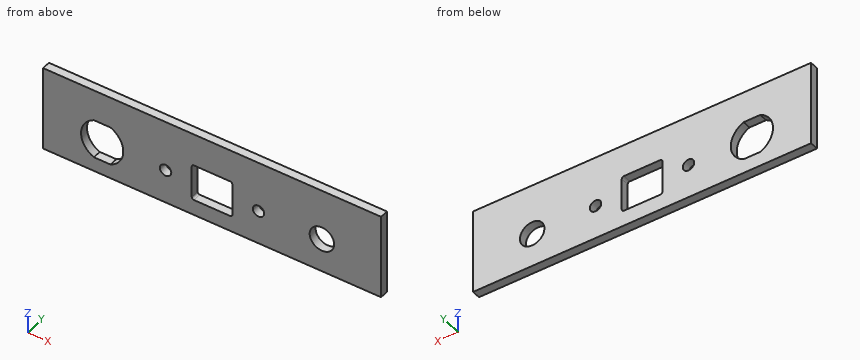
```python
from build123d import *

# Parameters (mm, degrees)
F0_W     = 101.6
F0_H     = 25.4
F1_DEPTH = 2.54
F2_R     = 1.7145
F2_R_2   = 3.683
F3_DEPTH = 2.541


with BuildPart() as f1:
    # F0 (on Front) → F1 (new body)
    with BuildSketch(Plane.XZ):
        with Locations((0, 2.54)):
            Rectangle(F0_W, F0_H)
    extrude(amount=-F1_DEPTH)

    # F2 (on face) → F3 (cut, through all)
    with BuildSketch(Plane.XZ):
        with BuildLine():
            Line((-30.531318, 5.842), (-35.508682, 5.842))
            ThreePointArc((-35.508682, 5.842), (-39.37, 0), (-35.508682, -5.842))
            Line((-35.508682, -5.842), (-30.531318, -5.842))
            ThreePointArc((-30.531318, -5.842), (-26.67, 0), (-30.531318, 5.842))
        make_face()
        with Locations((-13.97, 0)):
            Circle(F2_R)
        with Locations((13.97, 0)):
            Circle(F2_R)
        with Locations((33.02, 0)):
            Circle(F2_R_2)
        with BuildLine():
            ThreePointArc((6.096, 4.826), (5.910013, 5.275013), (5.461, 5.461))
            Line((5.461, 5.461), (-5.461, 5.461))
            ThreePointArc((-5.461, 5.461), (-5.910013, 5.275013), (-6.096, 4.826))
            Line((-6.096, 4.826), (-6.096, -4.826))
            ThreePointArc((-6.096, -4.826), (-5.910013, -5.275013), (-5.461, -5.461))
            Line((-5.461, -5.461), (5.461, -5.461))
            ThreePointArc((5.461, -5.461), (5.910013, -5.275013), (6.096, -4.826))
            Line((6.096, -4.826), (6.096, 4.826))
        make_face()
    extrude(amount=-F3_DEPTH, mode=Mode.SUBTRACT)


solid = f1.part
```
Source: CAD feature listing. Evaluate the final solid. Frame: model axes, mm. Give positions to 0.01 mm unless a question says otherwise; leave off trailing zeros. Loops run counter-clockwise (first coordinate to the right, second up) from the corner with the lowest first, then second, coordinate; pieces in that order, holes last. Notation, with made-up numbers: (-14, -30) -> (23, -30) arc R25 cw to (23, 6) -> close; hole circle Ø4 at (-9.75, 0.25). An arc over 180 degrees is marked (long way). Use a Markdown table: item, result. Add a question column.
(1) Section query C-C (y = 0.45). Count the separate pieces of the cut face and the enclosed holes in it, then the cut area to 3 significant figures.
(2) Ray query, line 1 (X direction, y = 1.95, z = -0.25); line 2 (Z direction, x = -33, y = 2.4); line 3 (Z direction, x = 13.97, y = 2.05). Return the intervals inside material, ascending.
(3) Section query A-A (x = 13.97). Output: boundary loops of the cut face in (y, z), then the cut area to 3 significant figures.
(4) Section query D-D (x = 33.02). Output: boundary loops of the cut face in (y, z), then the cut area to 3 significant figures.
(5) Section query B-B (z = 0). Output: boundary loops of the cut face in (x, y), then the cut area to 3 significant figures.
(6) First-contact query: pin 1 Ø4 at (x, z) = (-13.97, 0) entering from -Y. Flat tip, straight axial feed; report the tip coordinate or a pass-through.
Checked values:
| question | item | result |
|---|---|---|
| 1 | separate pieces | 1 |
| 1 | enclosed holes | 5 |
| 1 | area | 2,260 mm^2 |
| 2 | line 1 | -50.8 to -39.37, -26.67 to -15.67, -12.27 to -6.1, 6.1 to 12.27, 15.67 to 29.35, 36.69 to 50.8 |
| 2 | line 2 | -10.16 to -5.84, 5.84 to 15.24 |
| 2 | line 3 | -10.16 to -1.71, 1.71 to 15.24 |
| 3 | outline | (0, -10.16) -> (2.54, -10.16) -> (2.54, -1.71) -> (0, -1.71) -> close; (0, 1.71) -> (2.54, 1.71) -> (2.54, 15.24) -> (0, 15.24) -> close |
| 3 | area | 55.8 mm^2 |
| 4 | outline | (0, -10.16) -> (2.54, -10.16) -> (2.54, -3.68) -> (0, -3.68) -> close; (0, 3.68) -> (2.54, 3.68) -> (2.54, 15.24) -> (0, 15.24) -> close |
| 4 | area | 45.8 mm^2 |
| 5 | outline | (-50.8, 0) -> (-39.37, 0) -> (-39.37, 2.54) -> (-50.8, 2.54) -> close; (-26.67, 0) -> (-15.68, 0) -> (-15.68, 2.54) -> (-26.67, 2.54) -> close; (-12.26, 0) -> (-6.1, 0) -> (-6.1, 2.54) -> (-12.26, 2.54) -> close; (6.1, 0) -> (12.26, 0) -> (12.26, 2.54) -> (6.1, 2.54) -> close; (15.68, 0) -> (29.34, 0) -> (29.34, 2.54) -> (15.68, 2.54) -> close; (36.7, 0) -> (50.8, 0) -> (50.8, 2.54) -> (36.7, 2.54) -> close |
| 5 | area | 159 mm^2 |
| 6 | pin 1 | y = 0 |
